```python
from build123d import *

# Parameters (mm, degrees)
F0_W          = 445
F0_H          = 1084
F1_DEPTH      = 32
F3_DEPTH      = 10
F5_DEPTH      = 10
F7_DEPTH      = 22
F7_DEPTH_BACK = 10
F8_W          = 550
F8_H          = 29
F9_DEPTH      = 1189.001


with BuildPart() as f1:
    # F0 (on Front) → F1 (new body)
    with BuildSketch(Plane.XZ):
        Rectangle(F0_W, F0_H)
    extrude(amount=F1_DEPTH)

    # F2 (on face) → F3 (cut)
    with BuildSketch(Plane.XZ.offset(32)):
        Polygon((-19.5, -30), (-22.7926296995, -47.6978846347), (-5.0528002133, -50.7564759254), (78.1963408907, 396.7076575087), (60.5, 400), align=None)
        Polygon((222.5, -542), (222.5, -510), (190.5, -510), (-217.9259726344, -510), (-222.5, -512.0194736094), (-222.5, -542), align=None)
        Polygon((-145.1793725139, 213), (-148.2828207898, 195), (-185.2966065805, -19.6799575863), (-167.5583244971, -22.7382820834), (-164.5, -5), (-114.5, 285), (-132.2382820834, 288.0583244971), align=None)
        Polygon((-164.5, -5), (-167.5583244971, -22.7382820834), (-22.7926296995, -47.6978846347), (-19.5, -30), align=None)
        Polygon((-176.5, 213), (-176.5, 195), (-148.2828207898, 195), (-145.1793725139, 213), align=None)
        Polygon((-176.5, 510), (-194.5, 510), (-194.5, 195), (-176.5, 195), (-176.5, 213), (-176.5, 489.9562019444), align=None)
        Polygon((-81.6284831041, 50), (-26.3705931966, 510), (-44.5, 510), (-51.8361056045, 448.9298327582), (-54.11006781, 430), (-99.5, 52.1468311155), align=None)
        Polygon((-51.8361056045, 448.9298327582), (-176.5, 510), (-176.5, 489.9562019444), (-54.11006781, 430), align=None)
        Polygon((222.5, 542), (-222.5, 542), (-222.5, 510), (-194.5, 510), (-176.5, 510), (-44.5, 510), (-26.3705931966, 510), (190.5, 510), (222.5, 510), align=None)
        Polygon((222.5, -510), (222.5, 510), (190.5, 510), (190.5, -310), (190.5, -329.6763142865), (190.5, -510), align=None)
        Polygon((-222.5, -512.0194736094), (-222.5, -492.3431593229), (-366.9909259611, -556.1371833743), (-359.7208209674, -572.6036818904), align=None)
        Polygon((190.5, -310), (-222.5, -492.3431593229), (-222.5, -512.0194736094), (-217.9259726344, -510), (190.5, -329.6763142865), align=None)
    extrude(amount=-F3_DEPTH, mode=Mode.SUBTRACT)

    # F4 (on face) → F5 (cut, through all)
    with BuildSketch(Plane.XZ.offset(32)):
        Polygon((-222.5, 542), (-222.5, 506.7), (-197.8, 506.7), (-197.8, 191.7), (-152.2004758656, 191.7), (-189.109317787, -22.3712831437), (-2.4041469191, -54.5618298451), (82.0442661774, 399.3483905486), (57.8592669601, 403.8479252867), (-22.1486532942, -26.1946460803), (-160.6872887936, -2.3086744425), (-110.6872887936, 287.6913255575), (-134.9296076409, 291.8710357036), (-147.9590965553, 216.3), (-173.2, 216.3), (-173.2, 484.6649064346), (-57.665964291, 428.0672610853), (-103.1700304688, 49.2639720557), (-78.7456240443, 46.3299695312), (-23.4432839132, 506.7), (187.2, 506.7), (187.2, -307.8496549533), (-222.5, -488.7358350371), (-222.5, -542), (222.5, -542), (222.5, 542), align=None)
        Polygon((-202.2811579858, -506.7), (187.2, -334.7406178115), (187.2, -506.7), align=None, mode=Mode.SUBTRACT)
        Polygon((-54.5582159435, 453.9380325215), (-162.2623968703, 506.7), (-48.2201398778, 506.7), align=None, mode=Mode.SUBTRACT)
    extrude(amount=-F5_DEPTH, mode=Mode.SUBTRACT)

    # F6 (on face) → F7 (join, two sides)
    with BuildSketch(Plane.XZ.offset(22)) as f7_sk:
        with BuildLine():
            Line((-222.5, -192), (-222.5, -292))
            Line((-222.5, -292), (-265.1776695297, -334.6776695297))
            ThreePointArc((-265.1776695297, -334.6776695297), (-270.5969883128, -342.7882532502), (-272.5, -352.3553390593))
            Line((-272.5, -352.3553390593), (-272.5, -567))
            ThreePointArc((-272.5, -567), (-265.1776695297, -584.6776695297), (-247.5, -592))
            Line((-247.5, -592), (252.5, -592))
            ThreePointArc((252.5, -592), (270.1776695297, -584.6776695297), (277.5, -567))
            Line((277.5, -567), (277.5, 572))
            ThreePointArc((277.5, 572), (270.1776695297, 589.6776695297), (252.5, 597))
            Line((252.5, 597), (-247.5, 597))
            ThreePointArc((-247.5, 597), (-265.1776695297, 589.6776695297), (-272.5, 572))
            Line((-272.5, 572), (-272.5, -131.6446609407))
            ThreePointArc((-272.5, -131.6446609407), (-270.5969883128, -141.2117467498), (-265.1776695297, -149.3223304703))
            Line((-265.1776695297, -149.3223304703), (-222.5, -192))
        make_face()
        Polygon((-162.2623968703, 547), (-162.2623968703, 506.7), (-48.2201398778, 506.7), (-48.2201398778, 547), (192.5, 547), (192.5, 542), (222.5, 542), (222.5, 512), (227.5, 512), (227.5, 138.6296910943), (187.2, 138.6296910943), (187.2, 88.6296910943), (227.5, 88.6296910943), (227.5, -334.7406178115), (187.2, -334.7406178115), (187.2, -420.7203089057), (227.5, -420.7203089057), (227.5, -512), (222.5, -512), (222.5, -542), (192.5, -542), (192.5, -547), (-7.5405789929, -547), (-7.5405789929, -506.7), (-202.2811579858, -506.7), (-202.2811579858, -547), (-263.1881188044, -547), (-263.1881188044, -506.7), (-222.5, -488.7358350371), (-222.5, -398.0570733547), (-146.2218463421, -398.0570733547), (-146.2218463421, -83.5470482707), (-222.5, -83.5470482707), (-222.5, 547), align=None, mode=Mode.SUBTRACT)
    extrude(amount=-F7_DEPTH)
    extrude(f7_sk.sketch, amount=F7_DEPTH_BACK)

    # F8 (on face) → F9 (cut, through all)
    with BuildSketch(Plane.XY.offset(597)):
        with Locations((2.5, -14.5)):
            Rectangle(F8_W, F8_H)
    extrude(amount=-F9_DEPTH, mode=Mode.SUBTRACT)


solid = f1.part
```
Can you work these out from the model? Positions are in its coordinate system, mm. A direction names the side the tool comes from. Coordinates: 2 decimals unless noted, no trailing zeros. Loops run counter-clockwise (first coordinate to the right, second up) from the corner with the lowest first, then second, coordinate; pieces in that order, holes last. Notation, with made-up numbers: M -28.5,69 L 8.5,69 A28 cw 8.5,103 Z; hole C 59,27 d4. An arc over 180 degrees is marked long. Put each result on its own line as item: value. Start each with the question number.
(1) Imagine slicing it at D-D on y = -30.5. Give the number of separate pieces and of enclosed holes in the cut face, and give its area (3 significant figures).
(2) Which directions (+Z, -Z, +X, -X, +Y, -Y) give clear straight access to the entire face, cutting with the end or side of a thin tool? Please do faces 5 (the face through (-264.982, -30.479, 589.871)), 6 (the face through (-80.1, -30.5, 241.3)), 7 (the face through (-243.5, -30.5, -313)).
(3) I need wall thicknesses on probe 1 along Z at (x, y) = (219, -30.25); probe 2 along Z at (x, y) = (174, -29.3); probe 3 along X at (y, z) = (-31.75, -212.5). Which ranges of each line are inside material? Lowest first, please.
(4) Imagine slicing it at B-B on x = 9. List the corners of the cut face in (y, z) for me.
(5) Imagine slicing it at C-C on z = 152. List the corners of the cut face in (x, y) for me.
(6) We'd pull the mould along Z, two halves only. Please class faces 1 (the face through (-10.267, -30.521, -421.924)), 2 (the face through (-107.66, -30.52, 479.95)), 3 (the face through (-265.371, -30.479, -584.482)), 4 (the face through (60, -32, 11)): +Z half, -Z half, draft (parallel to the pull), parting line (faces both ways), or undercut.
(7) Imagine slicing it at A-A on z = -112.5. List the corners of the cut face in (x, y) for me, and give its area (3 significant figures).
Worked answers:
1. separate pieces: 1
1. enclosed holes: 3
1. area: 529,000 mm2
2. face 5: +Z, -X, +Y, -Y
2. face 6: +Y, -Y
2. face 7: -X, +Y, -Y
3. probe 1: z = -592 to -542, -420.72 to -334.74, 88.63 to 138.63, 542 to 597
3. probe 2: z = -592 to -547, -506.7 to -340.57, -313.68 to 506.7, 547 to 597
3. probe 3: x = -222.5 to 187.2, 227.5 to 277.5
4. outline: M -32,-592 L -29,-592 L -29,-547 L -32,-547 Z; M -32,-506.7 L -29,-506.7 L -29,-413.42 L -32,-413.42 Z; M -32,-386.53 L -29,-386.53 L -29,6.74 L -32,6.74 Z; M -32,141.23 L -29,141.23 L -29,506.7 L -32,506.7 Z; M -32,547 L -29,547 L -29,597 L -32,597 Z
5. outline: M -272.5,-32 L -159.05,-32 L -159.05,-29 L -272.5,-29 Z; M -134.08,-32 L -90.83,-32 L -90.83,-29 L -134.08,-29 Z; M -66.05,-32 L 11,-32 L 11,-29 L -66.05,-29 Z; M 36.03,-32 L 187.2,-32 L 187.2,-29 L 36.03,-29 Z; M 227.5,-32 L 277.5,-32 L 277.5,-29 L 227.5,-29 Z
6. face 1: undercut
6. face 2: undercut
6. face 3: -Z half
6. face 4: draft
7. outline: M -272.5,-32 L 187.2,-32 L 187.2,-29 L -272.5,-29 Z; M 227.5,-32 L 277.5,-32 L 277.5,-29 L 227.5,-29 Z
7. area: 1,530 mm2
